```python
from build123d import *

# Parameters (mm, degrees)
F1_DEPTH      = 50
F3_R          = 2.5796875
F4_DEPTH      = 17.146
F4_DEPTH_BACK = 9.526
F5_R          = 2.5796875
F5_R_2        = 9.525
F6_DEPTH      = 25.4


with BuildPart() as f1:
    # F0 (on Right) → F1 (new body)
    with BuildSketch(Plane.YZ):
        Polygon((22.1225786954, 25.4), (22.1225786954, -25.4), (48.7925786954, 38.1), align=None)
    extrude(amount=F1_DEPTH)

    # F3 (on offset) → F4 (cut, two sides)
    with BuildSketch(Plane.XZ.offset(-31.6475786954)) as f4_sk:
        with Locations((42.38, 17.78)):
            Circle(F3_R)
        with Locations((19.05, 17.78)):
            Circle(F3_R)
    extrude(amount=-F4_DEPTH, mode=Mode.SUBTRACT)
    extrude(f4_sk.sketch, amount=F4_DEPTH_BACK, mode=Mode.SUBTRACT)

    # F5 (on offset) → F6 (cut)
    with BuildSketch(Plane.XZ.offset(-31.6475786954)):
        with BuildLine():
            ThreePointArc((50, 12.065), (51.4162084139, 14.7679305287), (51.905, 17.78))
            ThreePointArc((51.905, 17.78), (51.4162084139, 20.7920694713), (50, 23.495))
            Line((50, 23.495), (50, 12.065))
        make_face()
        with BuildLine():
            Line((50, 12.065), (50, 23.495))
            ThreePointArc((50, 23.495), (32.855, 17.78), (50, 12.065))
        make_face()
        with Locations((42.38, 17.78)):
            Circle(F5_R, mode=Mode.SUBTRACT)
        with Locations((19.05, 17.78)):
            Circle(F5_R_2)
        with Locations((19.05, 17.78)):
            Circle(F5_R, mode=Mode.SUBTRACT)
    extrude(amount=-F6_DEPTH, mode=Mode.SUBTRACT)


solid = f1.part
```
Can you work these out from the model? Positions are in its coordinate system, mm. A direction names the side the tool comes from. Give positions to 0.01 mm unless a question says otherwise; leave off trailing zeros. Order: outer loops, then holes, each group sorted by start corner. A loop starts at its lowest first (then second) coordinate and runs counter-clockwise, first axis right, second up. Notation, with made-up numbers: (-1, 18.5) - (3, 18.5) arc R18 cw to (3, 52.5) - close; hole circle Ø2 at (-31.75, 13). An arc over 180 degrees is marked (long way). Use a Markdown table: item, result. Add a question column.
Q1. Please list where these lines run through material, in increasing order: line 1 along X through (y, z) = (25.75, 17.78); line 2 along X through (y, z) = (35.5, 17.78) (3 decimals); line 3 along Z through (x, y) = (19.05, 34) (3 decimals).
Q2. If we section it at B-B on z = 17.78: Write out the boundary of the cut face in (x, y) (3 decimals).
Q3. If we section it at A-A on x = 19.05: Write out the boundary of the cut face in (y, z) (3 decimals), plus the area to 3 significant figures.
Q4. On a 3-axis mill with a long thin cutter (end or side, diameter ignored), from which of +Z, -Z, +X, -X, +Y, -Y can I reach the whole of each face in a straight line? I mean faces 1 (the cylindrical face through (21.43, 26.95, 16.79)), 2 (the flat face through (21, 31.648, 15.8)). Say none if no direction works.
Q5. If we section it at D-D on x = 37: Write out the boundary of the cut face in (y, z).
Q6. I'm going to push flat-ended pins straight in: pin 1 (8 mm diameter, centred on x = 16.5, y = 36, fed in from +Z); pin 2 (1 mm diameter, centred on x = 14.5, z = 9.5, fed in from +Y); pin 3 (8.5 mm diameter, centred on x = 44, z = 21, fed in from +Y); pin 4 (4.5 mm diameter, centred on x = 19.05, z = 17.78, fed in from -Y). Where does each tip first touch, or does it pass through?
Q7. If we mould it in two halves opening along Z, with no side actions, what happens to faces 3 (the cylindrical face through (17.81, 36.464, 27.224)), 4 (the flat face through (24.65, 35.271, 5.906)), 5 (the cylindrical face through (44.76, 26.95, 16.79)), 6 (the flat face through (50, 30, 11))? For each: released by +Z, released by -Z, zero draft, split by the parting line, or undercut.
Q8. If we section it at C-C on y = 30: Write out the boundary of the cut face in (x, z).
Answers follow:
| question | item | result |
|---|---|---|
| 1 | line 1 | x = 0 to 16.47, 21.63 to 39.8, 44.96 to 50 |
| 1 | line 2 | x = 0 to 9.525, 28.575 to 32.855 |
| 1 | line 3 | z = 2.88 to 8.255, 27.305 to 31.056 |
| 2 | outline | (0, 22.123) - (16.47, 22.123) - (16.47, 31.648) - (9.525, 31.648) - (9.525, 40.258) - (0, 40.258) - close; (21.63, 22.123) - (39.8, 22.123) - (39.8, 31.648) - (32.855, 31.648) - (32.855, 40.258) - (28.575, 40.258) - (28.575, 31.648) - (21.63, 31.648) - close; (44.96, 22.123) - (50, 22.123) - (50, 31.648) - (44.96, 31.648) - close |
| 3 | outline | (22.123, -25.4) - (36.258, 8.255) - (31.648, 8.255) - (31.648, 15.2) - (22.123, 15.2) - close; (22.123, 20.36) - (31.648, 20.36) - (31.648, 27.305) - (44.259, 27.305) - (48.793, 38.1) - (22.123, 25.4) - close |
| 3 | area | 464 mm^2 |
| 4 | face 1 | +Y, -Y |
| 4 | face 2 | +Y |
| 5 | outline | (22.12, -25.4) - (36.96, 9.92) - (31.65, 9.92) - (31.65, 25.64) - (43.56, 25.64) - (48.79, 38.1) - (22.12, 25.4) - close |
| 6 | pin 1 | stops at z = 33.91 |
| 6 | pin 2 | stops at y = 36.86 |
| 6 | pin 3 | stops at y = 31.65 |
| 6 | pin 4 | passes through |
| 7 | face 3 | undercut |
| 7 | face 4 | released by -Z |
| 7 | face 5 | undercut |
| 7 | face 6 | zero draft |
| 8 | outline | (0, -6.64) - (50, -6.64) - (50, 29.15) - (0, 29.15) - close; hole circle Ø5.16 at (19.05, 17.78); hole circle Ø5.16 at (42.38, 17.78) |
